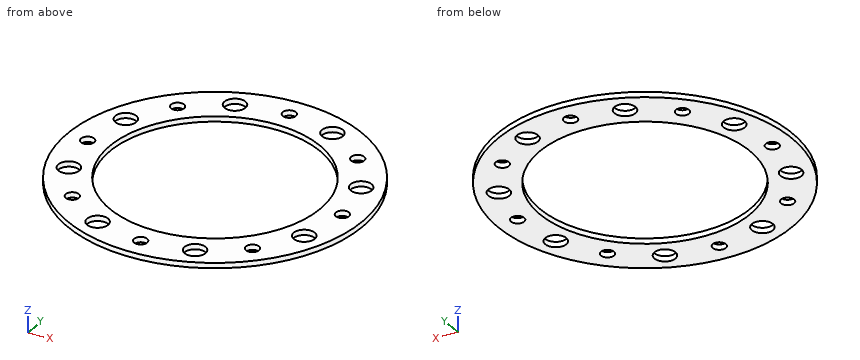
```python
from build123d import *

# Parameters (mm, degrees)
SKETCH1_R           = 28
SKETCH1_R_2         = 20
BOSS_EXTRUDE1_DEPTH = 1
CIRPATTERN1_COUNT   = 8
CIRPATTERN2_COUNT   = 8


with BuildPart() as part:
    # Sketch1 → Boss-Extrude1 (new body)
    with BuildSketch(Plane.XY):
        Circle(SKETCH1_R)
        Circle(SKETCH1_R_2, mode=Mode.SUBTRACT)
    extrude(amount=BOSS_EXTRUDE1_DEPTH)

    # Sketch2 → 2.5 _2.5_ Diameter Hole1 (revolve, cut)
    with BuildSketch(Plane(origin=(0, 24, 1), x_dir=(0, -1, 0), z_dir=(1, 0, 0))):
        Polygon((0, 0), (0, 2.251075774), (1.25, 1.5), (1.25, 0), align=None)
    f_2_5_2_5_diameter_hole1 = revolve(axis=Axis((0, 24, 7.35), (0, 0, -1)), mode=Mode.SUBTRACT)

    # CirPattern1: 2.5 _2.5_ Diameter Hole1 ×8 about axis
    cirpattern1_axis = Axis((0, 0, 0), (0, 0, 1))
    for i in range(1, CIRPATTERN1_COUNT):
        add(f_2_5_2_5_diameter_hole1.rotate(cirpattern1_axis, i * 360 / CIRPATTERN1_COUNT), mode=Mode.SUBTRACT)

    # Sketch4 → 4.0 _4_ Diameter Hole1 (revolve, cut)
    with BuildSketch(Plane(origin=(9.184402377, 22.17310878, 1), x_dir=(0, -1, 0), z_dir=(1, 0, 0))):
        Polygon((0, 0), (0, 2.701721238), (2, 1.5), (2, 0), align=None)
    f_4_0_4_diameter_hole1 = revolve(axis=Axis((9.184402377, 22.17310878, 7.35), (0, 0, -1)), mode=Mode.SUBTRACT)

    # CirPattern2: 4.0 _4_ Diameter Hole1 ×8 about axis
    cirpattern2_axis = Axis((0, 0, 0), (0, 0, 1))
    for i in range(1, CIRPATTERN2_COUNT):
        add(f_4_0_4_diameter_hole1.rotate(cirpattern2_axis, i * 360 / CIRPATTERN2_COUNT), mode=Mode.SUBTRACT)


solid = part.part
```
Here's how the part is built. I have some questions about the finished solid (model axes, mm). Round coordinates to 2 decimals unless told otherwise and drop trailing zeros. Write each loop counter-clockwise with the first axis right and the second up, starting at its lowest first coordinate (ties: lowest second). Pieces come first, ordered by that corner, then holes. Notation, with made-up numbers: M 2,3 L 6,3 A25 ccw 6,30 Z; hole C -38.5,83.25 d11. An arc over 180 degrees is marked long. Answer as CSV lines item,"result". Start each with the question number.
1. Suppose I cut it at D-D on y = 6. Write out the boundary of the cut face in (x, z), then the cut area to 3 significant figures.
2. I need wall thicknesses on probe 1 along Y at (x, z) = (0, 0.8); probe 2 along X at (y, z) = (17, 0.45); probe 3 along X at (y, z) = (-21.5, 0.4). Which ranges of each line are inside material? Lowest first, please.
3. I'm going to push a flat-ended pin straight in: pin 1 Ø3 at (x, y) = (-22.17, -9.18) entering from -Z. Where does the tip first touch, or does it pass through?
4. Suppose I cut it at C-C on z = 0.3. Count the separate pieces of the cut face and the enclosed holes in it, then the cut area to 3 significant figures.
5. Suppose I cut it at A-A on y = 0. Write out the boundary of the cut face in (x, z).
Check result:
1,outline,"M -27.35,0 L -19.08,0 L -19.08,1 L -27.35,1 Z; M 19.08,0 L 27.35,0 L 27.35,1 L 19.08,1 Z"
1,area,"16.5 mm2"
2,probe 1,"y = -28 to -25.25, -22.75 to -20, 20 to 22.75, 25.25 to 28"
2,probe 2,"x = -22.25 to -18.22, -15.72 to -10.54, 10.54 to 15.72, 18.22 to 22.25"
2,probe 3,"x = -17.94 to -11.07, -7.3 to 7.3, 11.07 to 17.94"
3,pin 1,"passes through"
4,separate pieces,"1"
4,enclosed holes,"17"
4,area,"1,070 mm2"
5,outline,"M -28,0 L -25.25,0 L -25.25,1 L -28,1 Z; M -22.75,0 L -20,0 L -20,1 L -22.75,1 Z; M 20,0 L 22.75,0 L 22.75,1 L 20,1 Z; M 25.25,0 L 28,0 L 28,1 L 25.25,1 Z"
